from build123d import *

# Parameters (mm, degrees)
EXTRUDE_1_DEPTH              = 2
SKETCH_2_R                   = 4.43
EXTRUDE_2_DEPTH              = 3.5
HOLE_WIZARD_M3_1_D           = 3.2
HOLE_WIZARD_M3_1_CSINK_D     = 6.3
HOLE_WIZARD_M3_1_CSINK_ANGLE = 90
SKETCH_8_R                   = 3
EXTRUDE_3_DEPTH              = 0.9
SKETCH_10_R                  = 1.52
CUT_EXTRUDE_1_DEPTH          = 2
CHAMFER_1_SIZE               = 0.2


with BuildPart() as part:
    # 草图1 → 凸台-拉伸1 (new body)
    with BuildSketch(Plane(origin=(0, 0, 12.16), x_dir=(-1, 0, 0), z_dir=(0, 0, -1))):
        with BuildLine():
            Line((10.90083304, -4.828267309), (11.334013857, -6.416349492))
            Line((11.334013857, -6.416349492), (12.2, -6.475))
            ThreePointArc((12.2, -6.475), (17.274650028, -4.0216355), (18.503750642, 1.479308233))
            ThreePointArc((18.503750642, 1.479308233), (18.045416815, 7.727850312), (19.542869864, 13.811597708))
            ThreePointArc((19.542869864, 13.811597708), (16.382825591, 19.863959761), (11.031173747, 15.624055427))
            ThreePointArc((11.031173747, 15.624055427), (10.022718521, 9.69776671), (7.334091643, 4.321042298))
            Line((7.334091643, 4.321042298), (8.685883448, 3.556822298))
            ThreePointArc((8.685883448, 3.556822298), (7.365813774, -1.276966534), (10.90083304, -4.828267309))
        make_face()
    extrude(amount=-EXTRUDE_1_DEPTH)

    # 草图2 → 凸台-拉伸2 (add)
    with BuildSketch(Plane(origin=(0, 0, 12.16), x_dir=(-1, 0, 0), z_dir=(0, 0, -1))):
        with Locations((15.460198425, 15.531101684)):
            Circle(SKETCH_2_R)
    extrude(amount=EXTRUDE_2_DEPTH)

    # M3 平头机械螺钉的锥形沉头孔1 (through all)
    with Locations(Plane.XY.offset(14.16)):
        with Locations((-15.5, 15.5)):
            CounterSinkHole(HOLE_WIZARD_M3_1_D / 2, HOLE_WIZARD_M3_1_CSINK_D / 2, counter_sink_angle=HOLE_WIZARD_M3_1_CSINK_ANGLE)

    # 草图8 → 凸台-拉伸3 (add)
    with BuildSketch(Plane(origin=(0, 0, 12.16), x_dir=(-1, 0, 0), z_dir=(0, 0, -1))):
        with Locations((12.24, 0)):
            Circle(SKETCH_8_R)
    extrude(amount=EXTRUDE_3_DEPTH)

    # 草图10 → 切除-拉伸1 (cut)
    with BuildSketch(Plane.XY.offset(11.26)):
        with Locations((-12.2, 0)):
            Circle(SKETCH_10_R)
    extrude(amount=CUT_EXTRUDE_1_DEPTH, mode=Mode.SUBTRACT)

    # 倒角1
    chamfer_1_edges = [part.edges().sort_by_distance(p)[0] for p in [
        (-16.382825591, 19.863959761, 14.16),
        (-10.022718521, 9.69776671, 14.16),
        (-8.009987545, 3.938932298, 14.16),
        (-7.365813774, -1.276966534, 14.16),
        (-11.117423449, -5.622308401, 14.16),
        (-11.767006928, -6.445674746, 14.16),
        (-17.274650028, -4.0216355, 14.16),
        (-18.045416815, 7.727850312, 14.16),
    ]]
    chamfer(chamfer_1_edges, length=CHAMFER_1_SIZE)


solid = part.part
Source: CAD feature listing. Evaluate the final solid. Frame: model axes, mm. A direction names the side the tool comes from. Round coordinates to 2 decimals unless told otherwise and drop trailing zeros. Loops run counter-clockwise (first coordinate to the right, second up) from the corner with the lowest first, then second, coordinate; pieces in that order, holes last.
Q1. Section A-A, the plane y = 0. Return loops of the section in (x, z) (3 decimals).
Q2. Ray query, line 1 (X direction, y = 15.5, z = 11.05); line 2 (Y direction, x = -15.5, z = 9.65); line 3 (Y direction, x = -14.5, z = 11.55). Return the intervals inside material, ascending.
Q3. First-contact query: P1, Ø3, axis at x = -13, z = 11.5, coming from the +Y side; P2, Ø0.9, axis at x = -12, y = -0.5, coming from the -Z side; P3, Ø3, axis at x = -13, y = -0.5, coming from the -Z side. Flat tips, straight axial feed; report the tip coordinate or a pass-through.
Q4. Mould query, pull axis X, two halves, no side actions, for faces 1 (the face through (-12, 0, 13.26)), 2 (the face through (-13.72, 0.07, 12.25)), 3 (the face through (-10.05, 9.78, 13.05)), 4 (the face through (-13, 5, 12.16)). Classes: pulls with the +X half, pulls with the -X half, needs draft (parallel to the pull), parting line crosses it, or undercut.
Q5. Section B-B, the plane z = 10.35. Return loops of the section in (x, y).
Q6. Access query for faces 5 (the face through (-8.001, 3.944, 13.047)), 6 (the face through (-13, 4, 14.16)), 7 (the face through (-14, -1, 11.26)), 8 (the face through (-17.4, 15.6, 8.66)), 9 (the face through (-9.243, 0.132, 11.716)). Directions: +Z, -Z, +X, -X, +Y, -Y. A direction counts if a zero-diameter tool reaches every point of the face in a straight line with its end or side. Return the directions, or none.
Solutions:
1. outline: (-18.675, 12.16) - (-15.24, 12.16) - (-15.24, 11.26) - (-13.72, 11.26) - (-13.72, 13.26) - (-10.68, 13.26) - (-10.68, 11.26) - (-9.24, 11.26) - (-9.24, 12.16) - (-7.2, 12.16) - (-7.2, 13.96) - (-7.4, 14.16) - (-18.475, 14.16) - (-18.675, 13.96) - close
2. line 1: x = -19.89 to -17.1, -13.9 to -11.03
2. line 2: y = 11.1 to 13.9, 17.1 to 19.96
2. line 3: y = -1.97 to 1.97, 11.21 to 14.25, 16.75 to 19.86
3. P1: stops at y = 19.86
3. P2: stops at z = 13.26
3. P3: stops at z = 11.26
4. face 1: undercut
4. face 2: undercut
4. face 3: pulls with the +X half
4. face 4: needs draft
5. outline: circle Ø8.86 at (-15.46, 15.53); hole circle Ø3.2 at (-15.5, 15.5)
6. face 5: +Z, -Z, +X
6. face 6: +Z, +X, -X, +Y, -Y
6. face 7: -Z, +X, -X, -Y
6. face 8: -Z, +X, -X, +Y, -Y
6. face 9: -Z
